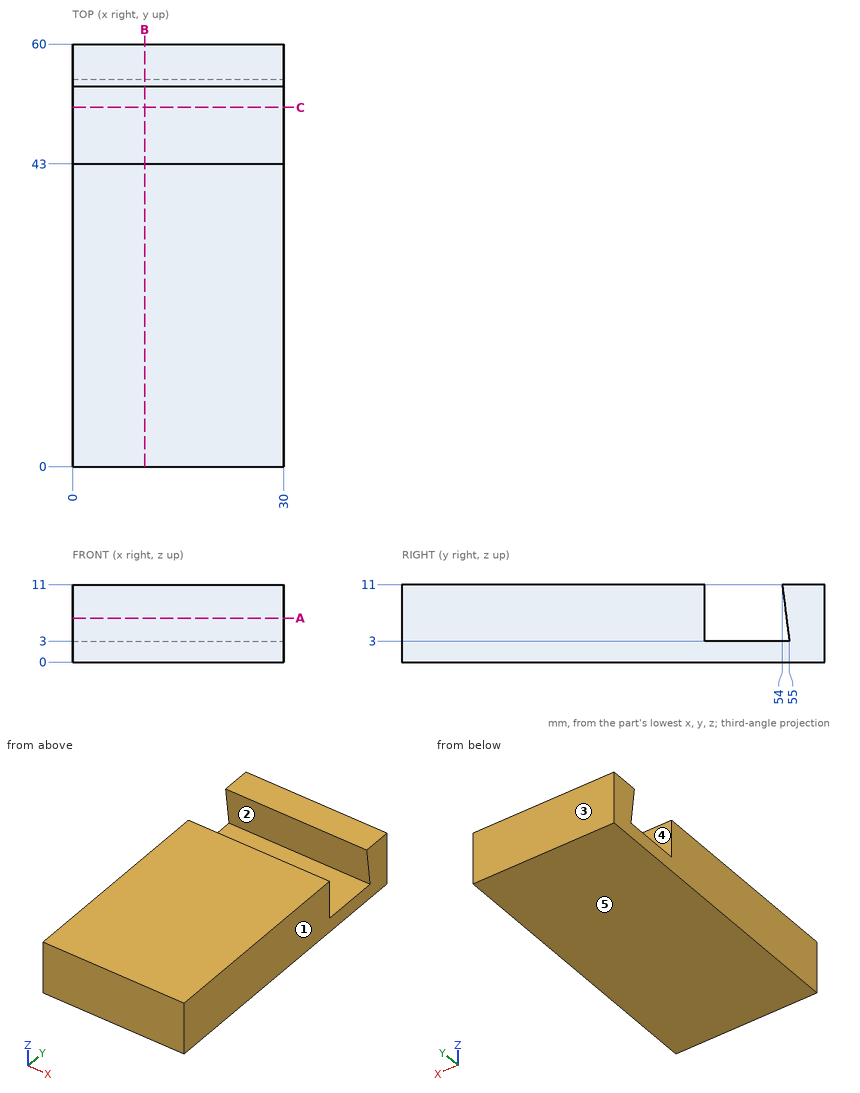
Can you work these out from the drawing? Everything is in mm from the part's minimum corner. A direction names the side the tool comes from. Give positions to 0.01 mm unless a question says otherwise; leave off trailing zeros. Loops run counter-clockwise (first coordinate to the right, second up) from the corner with the lowest first, then second, coordinate; pieces in that order, holes last. Notation, with made-up numbers: (74, 86.5) -> (133, 86.5) arc R24 cw to (133, 105.5) -> close; hole circle Ø8 at (22.25, -28.5). An arc over 180 degrees is marked (long way). Put each result on its own line as item: value.
(1) Please list where these lines run through material, in increasing order: probe 1 along Z at (x, y) = (12, 46.5); probe 2 along Y at (x, z) = (22.5, 6) (3 decimals); probe 3 along Y at (x, z) = (12, 4.75). Write a range as [from, to].
Computed:
probe 1: [0, 3]
probe 2: [0, 43], [54.625, 60]
probe 3: [0, 43], [54.78, 60]
(2) Imagine slicing it at C-C on y = 51. Write out the boundary of the cut face in (x, z).
Computed:
outline: (0, 0) -> (30, 0) -> (30, 3) -> (0, 3) -> close
(3) Thinking about a two-plate mould opening in Y: for the marked faces 3, 4 and 5, which applies, pulls with the +Y half, pulls with the -Y half, needs draft (parallel to the pull), parting line crosses it, or undercut?
Computed:
face 3: pulls with the +Y half
face 4: undercut
face 5: needs draft
(4) I'm going to push a flat-ended pin straight in: pin 1 Ø3 at (x, y) = (3.5, 51) entering from +Z. Where does the tip first touch, or does it pass through?
Computed:
pin 1: z = 3
(5) Imagine slicing it at B-B on x = 10.25. Write out the boundary of the cut face in (y, z).
Computed:
outline: (0, 0) -> (60, 0) -> (60, 11) -> (54, 11) -> (55, 3) -> (43, 3) -> (43, 11) -> (0, 11) -> close
(6) Imagine slicing it at A-A on z = 6.25. Write out the boundary of the cut face in (x, y), plus the area to 3 significant figures.
Computed:
outline: (0, 0) -> (30, 0) -> (30, 43) -> (0, 43) -> close; (0, 54.59) -> (30, 54.59) -> (30, 60) -> (0, 60) -> close
area: 1,450 mm^2
(7) For the marked faces 1 and 2, which set-ups out of +Z, -Z, +X, -X, +Y, -Y let a thin tool reach every point of the face, with its end or its side?
Computed:
face 1: +Z, -Z, +X, +Y, -Y
face 2: +X, -X
